Here's how the part is built. I have some questions about the finished solid (model axes, mm). A direction names the side the tool comes from. Round coordinates to 2 decimals unless told otherwise and drop trailing zeros. Order: outer loops, then holes, each group sorted by start corner. A loop starts at its lowest first (then second) coordinate and runs counter-clockwise, first axis right, second up.
```python
from build123d import *

# Parameters (mm, degrees)
EXTRUDE_1_DEPTH           = 3
CUT_EXTRUDE_1_REACH       = 127.841
FILLET_1_R                = 3
FILLET_3_R                = 3
CUT_EXTRUDE_2_REACH       = 127.841
SKETCH_3_R                = 1.6
FILLET_4_R                = 2
CUT_EXTRUDE_4_REACH       = 127.841
SKETCH_5_R                = 1.6
CUT_EXTRUDE_5_REACH       = 127.841
SKETCH_6_R                = 2.25
HOLE_WIZARD_1_D           = 3.4
HOLE_WIZARD_1_DEPTH       = 3
HOLE_WIZARD_1_CSINK_D     = 6.6
HOLE_WIZARD_1_CSINK_ANGLE = 90
HOLE_WIZARD_1_TIP         = 1.021463052
CUT_EXTRUDE_6_REACH       = 127.841
SKETCH_9_R                = 1.6
SKETCH_10_R               = 107.153913746
SKETCH_10_R_2             = 87
CUT_EXTRUDE_7_DEPTH       = 10
FILLET_5_R                = 3
SKETCH_12_W               = 2.492222484
SKETCH_12_H               = 8
CUT_EXTRUDE_8_DEPTH       = 10
FILLET_6_R                = 1
FILLET_7_R                = 3
HOLE_WIZARD_2_D           = 3.4
HOLE_WIZARD_2_DEPTH       = 3
HOLE_WIZARD_2_CSINK_D     = 6.6
HOLE_WIZARD_2_CSINK_ANGLE = 90
HOLE_WIZARD_2_TIP         = 1.021463052
HOLE_WIZARD_3_D           = 2.9
HOLE_WIZARD_3_DEPTH       = 3
HOLE_WIZARD_3_CSINK_D     = 5.4
HOLE_WIZARD_3_CSINK_ANGLE = 90
HOLE_WIZARD_3_TIP         = 0.871247898
CUT_EXTRUDE_10_DEPTH      = 10
FILLET_8_R                = 1
SKETCH1_R                 = 1.6
EXTRUDE1_DEPTH            = 10


with BuildPart() as part:
    # 草图1 → 凸台-拉伸1 (new body)
    with BuildSketch(Plane.XY):
        with BuildLine():
            Line((-45, 40.484634583), (-47.790898075, 55.614169672))
            Line((-47.790898075, 55.614169672), (-71.258078067, 18.058831232))
            Line((-71.258078067, 18.058831232), (-85.105103955, 26.040761909))
            ThreePointArc((-85.105103955, 26.040761909), (-87.951877875, -13.618633494), (-73.244121351, -50.559852526))
            Line((-73.244121351, -50.559852526), (-60.839609095, -38.155340271))
            Line((-60.839609095, -38.155340271), (-36.030129611, -62.964819755))
            Line((-36.030129611, -62.964819755), (-48.007288857, -74.941979001))
            ThreePointArc((-48.007288857, -74.941979001), (-38.539553852, -80.222832092), (-28.5, -84.313403442))
            Line((-28.5, -84.313403442), (-28.5, -46.350874392))
            Line((-28.5, -46.350874392), (-10, -46.350874392))
            Line((-10, -46.350874392), (-10, -88.350874392))
            ThreePointArc((-10, -88.350874392), (-5.007949588, -88.773855648), (0, -88.914998767))
            Line((0, -88.914998767), (0, 40.484634583))
            Line((0, 40.484634583), (-45, 40.484634583))
        make_face()
    extrude(amount=EXTRUDE_1_DEPTH)

    # 草图2 → 切除-拉伸1 (cut, up to next)
    with BuildSketch(Plane.XY.offset(3), mode=Mode.PRIVATE) as cut_extrude_1_sk1:
        Polygon((-12, 0), (-12, 30), (-52, 30), (-69.320508076, 0), (-66.769463395, -15.795321176), (-36.939246535, -45.625538036), (-26.313708499, -35), (-12, -35), align=None)
    cut_extrude_1_tool1 = extrude(cut_extrude_1_sk1.sketch, amount=-CUT_EXTRUDE_1_REACH, mode=Mode.PRIVATE) & part.part
    add(cut_extrude_1_tool1.solids().sort_by_distance((-37.08097, -3.648282, 3))[0], mode=Mode.SUBTRACT)

    # 圆角1
    fillet_1_edges = [part.edges().sort_by_distance(p)[0] for p in [
        (-71.258078067, 18.058831232, 1.5),
        (-45, 40.484634583, 1.5),
        (-36.030129611, -62.964819755, 1.5),
        (-60.839609095, -38.155340271, 1.5),
    ]]
    fillet(fillet_1_edges, radius=FILLET_1_R)

    # 圆角3
    fillet_3_edges = [part.edges().sort_by_distance(p)[0] for p in [
        (-66.769463395, -15.795321176, 1.5),
        (-69.320508076, 0, 1.5),
        (-52, 30, 1.5),
        (-12, 30, 1.5),
        (-12, -35, 1.5),
        (-26.313708499, -35, 1.5),
        (-36.939246535, -45.625538036, 1.5),
    ]]
    fillet(fillet_3_edges, radius=FILLET_3_R)

    # 镜向2: part across plane


with BuildPart() as part_1:
    add(part.part)
    add(part.part.mirror(Plane(origin=(0, 40.484634583, 3), x_dir=(0, 0, 1), z_dir=(-1, 0, 0))))

    # 草图3 → 切除-拉伸2 (cut, up to next)
    with BuildSketch(Plane.XY.offset(3), mode=Mode.PRIVATE) as cut_extrude_2_sk1:
        with Locations((-81.739855024, -13.201505688)):
            Circle(SKETCH_3_R)
    cut_extrude_2_tool1 = extrude(cut_extrude_2_sk1.sketch, amount=-CUT_EXTRUDE_2_REACH, mode=Mode.PRIVATE) & part_1.part
    # 草图3 → 切除-拉伸2 (cut, up to next)
    with BuildSketch(Plane.XY.offset(3), mode=Mode.PRIVATE) as cut_extrude_2_sk2:
        with Locations((0, -36.25)):
            Circle(SKETCH_3_R)
    cut_extrude_2_tool2 = extrude(cut_extrude_2_sk2.sketch, amount=-CUT_EXTRUDE_2_REACH, mode=Mode.PRIVATE) & part_1.part
    # 草图3 → 切除-拉伸2 (cut, up to next)
    with BuildSketch(Plane.XY.offset(3), mode=Mode.PRIVATE) as cut_extrude_2_sk3:
        with Locations((0, 25)):
            Circle(SKETCH_3_R)
    cut_extrude_2_tool3 = extrude(cut_extrude_2_sk3.sketch, amount=-CUT_EXTRUDE_2_REACH, mode=Mode.PRIVATE) & part_1.part
    # 草图3 → 切除-拉伸2 (cut, up to next)
    with BuildSketch(Plane.XY.offset(3), mode=Mode.PRIVATE) as cut_extrude_2_sk4:
        with Locations((81.739855024, -13.201505688)):
            Circle(SKETCH_3_R)
    cut_extrude_2_tool4 = extrude(cut_extrude_2_sk4.sketch, amount=-CUT_EXTRUDE_2_REACH, mode=Mode.PRIVATE) & part_1.part
    add(cut_extrude_2_tool1.solids().sort_by_distance((-81.739855, -13.201506, 3))[0], mode=Mode.SUBTRACT)
    add(cut_extrude_2_tool2.solids().sort_by_distance((0, -36.25, 3))[0], mode=Mode.SUBTRACT)
    add(cut_extrude_2_tool3.solids().sort_by_distance((0, 25, 3))[0], mode=Mode.SUBTRACT)
    add(cut_extrude_2_tool4.solids().sort_by_distance((81.739855, -13.201506, 3))[0], mode=Mode.SUBTRACT)

    # 圆角4
    fillet_4_edges = [part_1.edges().sort_by_distance(p)[0] for p in [
        (47.790898075, 55.614169672, 1.5),
        (-47.790898075, 55.614169672, 1.5),
    ]]
    fillet(fillet_4_edges, radius=FILLET_4_R)

    # 草图5 → 切除-拉伸4 (cut, up to next)
    with BuildSketch(Plane.XY.offset(3), mode=Mode.PRIVATE) as cut_extrude_4_sk1:
        with Locations((-4, 34.39963335)):
            Circle(SKETCH_5_R)
    cut_extrude_4_tool1 = extrude(cut_extrude_4_sk1.sketch, amount=-CUT_EXTRUDE_4_REACH, mode=Mode.PRIVATE) & part_1.part
    # 草图5 → 切除-拉伸4 (cut, up to next)
    with BuildSketch(Plane.XY.offset(3), mode=Mode.PRIVATE) as cut_extrude_4_sk2:
        with Locations((4, 34.39963335)):
            Circle(SKETCH_5_R)
    cut_extrude_4_tool2 = extrude(cut_extrude_4_sk2.sketch, amount=-CUT_EXTRUDE_4_REACH, mode=Mode.PRIVATE) & part_1.part
    add(cut_extrude_4_tool1.solids().sort_by_distance((-4, 34.399633, 3))[0], mode=Mode.SUBTRACT)
    add(cut_extrude_4_tool2.solids().sort_by_distance((4, 34.399633, 3))[0], mode=Mode.SUBTRACT)

    # 草图6 → 切除-拉伸5 (cut, up to next)
    with BuildSketch(Plane.XY.offset(3), mode=Mode.PRIVATE) as cut_extrude_5_sk1:
        with Locations((-75, -23)):
            Circle(SKETCH_6_R)
    cut_extrude_5_tool1 = extrude(cut_extrude_5_sk1.sketch, amount=-CUT_EXTRUDE_5_REACH, mode=Mode.PRIVATE) & part_1.part
    # 草图6 → 切除-拉伸5 (cut, up to next)
    with BuildSketch(Plane.XY.offset(3), mode=Mode.PRIVATE) as cut_extrude_5_sk2:
        with Locations((75, -23)):
            Circle(SKETCH_6_R)
    cut_extrude_5_tool2 = extrude(cut_extrude_5_sk2.sketch, amount=-CUT_EXTRUDE_5_REACH, mode=Mode.PRIVATE) & part_1.part
    add(cut_extrude_5_tool1.solids().sort_by_distance((-75, -23, 3))[0], mode=Mode.SUBTRACT)
    add(cut_extrude_5_tool2.solids().sort_by_distance((75, -23, 3))[0], mode=Mode.SUBTRACT)

    # 打孔尺寸(%根据十字)槽沉头木螺钉的类型1
    with Locations(Plane(origin=(-69.5, 13, 3), x_dir=(1, 0, 0), z_dir=(0, 0, 1))):
        with Locations((0, 0), (3.5, -38), (139, 0), (135.5, -38)):
            CounterSinkHole(HOLE_WIZARD_1_D / 2, HOLE_WIZARD_1_CSINK_D / 2, depth=HOLE_WIZARD_1_DEPTH, counter_sink_angle=HOLE_WIZARD_1_CSINK_ANGLE)
            with Locations((0, 0, -(HOLE_WIZARD_1_DEPTH + HOLE_WIZARD_1_TIP / 2))):  # 118° drill point
                Cone(0, HOLE_WIZARD_1_D / 2, HOLE_WIZARD_1_TIP, mode=Mode.SUBTRACT)

    # 草图9 → 切除-拉伸6 (cut, up to next)
    with BuildSketch(Plane.XY.offset(3), mode=Mode.PRIVATE) as cut_extrude_6_sk1:
        with Locations((-48.412128424, 43.22221775)):
            Circle(SKETCH_9_R)
    cut_extrude_6_tool1 = extrude(cut_extrude_6_sk1.sketch, amount=-CUT_EXTRUDE_6_REACH, mode=Mode.PRIVATE) & part_1.part
    # 草图9 → 切除-拉伸6 (cut, up to next)
    with BuildSketch(Plane.XY.offset(3), mode=Mode.PRIVATE) as cut_extrude_6_sk2:
        with Locations((-35.355339059, -55.154328933)):
            Circle(SKETCH_9_R)
    cut_extrude_6_tool2 = extrude(cut_extrude_6_sk2.sketch, amount=-CUT_EXTRUDE_6_REACH, mode=Mode.PRIVATE) & part_1.part
    # 草图9 → 切除-拉伸6 (cut, up to next)
    with BuildSketch(Plane.XY.offset(3), mode=Mode.PRIVATE) as cut_extrude_6_sk3:
        with Locations((48.412128424, 43.22221775)):
            Circle(SKETCH_9_R)
    cut_extrude_6_tool3 = extrude(cut_extrude_6_sk3.sketch, amount=-CUT_EXTRUDE_6_REACH, mode=Mode.PRIVATE) & part_1.part
    # 草图9 → 切除-拉伸6 (cut, up to next)
    with BuildSketch(Plane.XY.offset(3), mode=Mode.PRIVATE) as cut_extrude_6_sk4:
        with Locations((35.355339059, -55.154328933)):
            Circle(SKETCH_9_R)
    cut_extrude_6_tool4 = extrude(cut_extrude_6_sk4.sketch, amount=-CUT_EXTRUDE_6_REACH, mode=Mode.PRIVATE) & part_1.part
    add(cut_extrude_6_tool1.solids().sort_by_distance((-48.412128, 43.222218, 3))[0], mode=Mode.SUBTRACT)
    add(cut_extrude_6_tool2.solids().sort_by_distance((-35.355339, -55.154329, 3))[0], mode=Mode.SUBTRACT)
    add(cut_extrude_6_tool3.solids().sort_by_distance((48.412128, 43.222218, 3))[0], mode=Mode.SUBTRACT)
    add(cut_extrude_6_tool4.solids().sort_by_distance((35.355339, -55.154329, 3))[0], mode=Mode.SUBTRACT)

    # 草图10 → 切除-拉伸7 (cut)
    with BuildSketch(Plane.XY.offset(3)):
        Circle(SKETCH_10_R)
        Circle(SKETCH_10_R_2, mode=Mode.SUBTRACT)
    extrude(amount=-CUT_EXTRUDE_7_DEPTH, mode=Mode.SUBTRACT)

    # 圆角5
    fillet_5_edges = [part_1.edges().sort_by_distance(p)[0] for p in [
        (83.326083977, 25.015269919, 1.5),
        (-71.80580935, -49.121540525, 1.5),
        (-46.558737732, -73.493427875, 1.5),
        (46.558737732, -73.493427875, 1.5),
        (71.80580935, -49.121540525, 1.5),
        (-83.326083977, 25.015269919, 1.5),
    ]]
    fillet(fillet_5_edges, radius=FILLET_5_R)

    # 草图12 → 切除-拉伸8 (cut)
    with BuildSketch(Plane.XY.offset(3)):
        with Locations((-86.746111242, 0)):
            Rectangle(SKETCH_12_W, SKETCH_12_H)
        with Locations((86.746111242, 0)):
            Rectangle(SKETCH_12_W, SKETCH_12_H)
    extrude(amount=-CUT_EXTRUDE_8_DEPTH, mode=Mode.SUBTRACT)

    # 圆角6
    fillet_6_edges = [part_1.edges().sort_by_distance(p)[0] for p in [
        (-85.5, 4, 1.5),
        (-85.5, -4, 1.5),
        (85.5, -4, 1.5),
        (85.5, 4, 1.5),
    ]]
    fillet(fillet_6_edges, radius=FILLET_6_R)

    # 圆角7
    fillet_7_edges = [part_1.edges().sort_by_distance(p)[0] for p in [
        (28.5, -46.350874392, 1.5),
        (10, -46.350874392, 1.5),
        (-10, -46.350874392, 1.5),
        (-28.5, -46.350874392, 1.5),
        (-28.5, -82.199452553, 1.5),
        (-10, -86.423376467, 1.5),
        (10, -86.423376467, 1.5),
        (28.5, -82.199452553, 1.5),
    ]]
    fillet(fillet_7_edges, radius=FILLET_7_R)

    # 打孔尺寸(%根据十字)槽沉头木螺钉的类型2
    with Locations(Plane(origin=(0, -49, 3), x_dir=(1, 0, 0), z_dir=(0, 0, 1))):
        with Locations((0, 0), (0, -29)):
            CounterSinkHole(HOLE_WIZARD_2_D / 2, HOLE_WIZARD_2_CSINK_D / 2, depth=HOLE_WIZARD_2_DEPTH, counter_sink_angle=HOLE_WIZARD_2_CSINK_ANGLE)
            with Locations((0, 0, -(HOLE_WIZARD_2_DEPTH + HOLE_WIZARD_2_TIP / 2))):  # 118° drill point
                Cone(0, HOLE_WIZARD_2_D / 2, HOLE_WIZARD_2_TIP, mode=Mode.SUBTRACT)

    # 打孔尺寸(%根据十字)槽沉头木螺钉的类型3
    with Locations(Plane(origin=(-6, -64.696867821, 3), x_dir=(1, 0, 0), z_dir=(0, 0, 1))):
        with Locations((0, 0), (12, 0)):
            CounterSinkHole(HOLE_WIZARD_3_D / 2, HOLE_WIZARD_3_CSINK_D / 2, depth=HOLE_WIZARD_3_DEPTH, counter_sink_angle=HOLE_WIZARD_3_CSINK_ANGLE)
            with Locations((0, 0, -(HOLE_WIZARD_3_DEPTH + HOLE_WIZARD_3_TIP / 2))):  # 118° drill point
                Cone(0, HOLE_WIZARD_3_D / 2, HOLE_WIZARD_3_TIP, mode=Mode.SUBTRACT)

    # 草图17 → 切除-拉伸10 (cut)
    with BuildSketch(Plane.XY.offset(3)):
        Polygon((-28.5, -84.313403442), (-28.5, -74.313403442), (-35.708850961, -81.522254403), align=None)
        Polygon((35.708850961, -81.522254403), (28.5, -84.313403442), (28.5, -74.313403442), align=None)
    extrude(amount=-CUT_EXTRUDE_10_DEPTH, mode=Mode.SUBTRACT)

    # 圆角8
    fillet_8_edges = [part_1.edges().sort_by_distance(p)[0] for p in [
        (-34.18780779, -80.001211232, 1.5),
        (-28.5, -74.313403442, 1.5),
        (34.18780779, -80.001211232, 1.5),
        (28.5, -74.313403442, 1.5),
    ]]
    fillet(fillet_8_edges, radius=FILLET_8_R)

    # Sketch1 → Extrude1 (cut)
    with BuildSketch(Plane.XY.offset(3)):
        with Locations((24.5, 35.484634583)):
            Circle(SKETCH1_R)
        with Locations((-24.5, 35.484634583)):
            Circle(SKETCH1_R)
    extrude(amount=-EXTRUDE1_DEPTH, mode=Mode.SUBTRACT)


solid = part_1.part
```
1) I'm going to push flat-ended pins straight in: pin 1 (0.9 mm diameter, centred on y = -65, z = 1.5, fed in from -X); pin 2 (4 mm diameter, centred on x = 4, y = 34.4, fed in from +Z); pin 3 (0.9 mm diameter, centred on x = -17.5, z = 2, fed in from -Y); pin 4 (1.5 mm diameter, centred on x = 42, z = 2, fed in from -Y). Where does each tip first touch, or does it pass through?
2) I need wall thicknesses on line 1 (X direction, y = -53.5, z = 1.7); line 2 (Y direction, x = -4, z = 0.7); line 3 (X direction, y = -7, z = 0.65). Which ranges of each line are inside material? Lowest first, please.
3) For faces 1 (the cylindrical face through (39.014, -77.762, 1.521)), 2 (the flat face through (-31.216, -77.029, 1.521)), 3 (the flat face through (48.579, -50.416, 1.479)), which set-ups out of +Z, -Z, +X, -X, +Y, -Y let a thin tool reach every point of the face, with its end or its side?
4) If we section it at A-A (x = -18): Write out the boundary of the cut face in (y, z), plus the area to 3 significant figures.
5) If we section it at B-B (y = -7.5): Write out the boundary of the cut face in (x, z).
6) We'd pull the mould along X, two halves only. Please class faces 4 (the flat face through (40.96, -67.894, 1.479)), 5 (the flat face through (-66.121, -43.436, 1.479)), 6 (the cylindrical face through (-83.17, -25.53, 1.52)), 7 (the cylindrical face through (-73.962, -24.996, 1.521)): +X half, -X half, draft (parallel to the pull), parting line (faces both ways), or undercut.
Solutions:
1. pin 1: stops at x = -38.52
1. pin 2: stops at z = 3
1. pin 3: stops at y = -46.35
1. pin 4: stops at y = -76.6
2. line 1: x = -45.49 to -28.5, -10 to 10, 28.5 to 45.49
2. line 2: y = -86.91 to 32.8, 36 to 40.48
2. line 3: x = -86.72 to -68.19, -12 to 12, 68.19 to 86.72
3. face 1: +Z, -Z, +X, -Y
3. face 2: +Z, -Z, -Y
3. face 3: +Z, -Z
4. outline: (-46.35, 0) - (-35, 0) - (-35, 3) - (-46.35, 3) - close; (30, 0) - (40.48, 0) - (40.48, 3) - (30, 3) - close
4. area: 65.5 mm2
5. outline: (-86.68, 0) - (-68.11, 0) - (-68.11, 3) - (-86.68, 3) - close; (-12, 0) - (12, 0) - (12, 3) - (-12, 3) - close; (68.11, 0) - (86.68, 0) - (86.68, 3) - (68.11, 3) - close
6. face 4: +X half
6. face 5: undercut
6. face 6: -X half
6. face 7: undercut
